The listing builds one solid part. Answer for the finished solid, in the listing's coordinates (mm). A direction names the side the tool comes from. Give positions to 0.01 mm unless a question says otherwise; leave off trailing zeros. Order: outer loops, then holes, each group sorted by start corner. A loop starts at its lowest first (then second) coordinate and runs counter-clockwise, first axis right, second up. Notation, with made-up numbers: M 53,-36 L 103,-36 A22 ccw 103,0 Z; hole C -25,22 d9. An arc over 180 degrees is marked long. Answer as a JSON object with one key per item and string values. Group by question number.
```python
from build123d import *

# Parameters (mm, degrees)
BOSS_EXTRUDE1_DEPTH = 6
CUT_EXTRUDE1_DEPTH  = 2.5
SKETCH3_R           = 1
CUT_EXTRUDE2_DEPTH  = 7
SKETCH4_R           = 2
CUT_EXTRUDE3_DEPTH  = 1.5
SKETCH5_R           = 1.25
CUT_EXTRUDE4_DEPTH  = 7


with BuildPart() as part:
    # Sketch1 → Boss-Extrude1 (new body)
    with BuildSketch(Plane.XY):
        with BuildLine():
            Line((0, 4.5), (23, 4.5))
            ThreePointArc((23, 4.5), (27.5, 0), (23, -4.5))
            Line((23, -4.5), (0, -4.5))
            ThreePointArc((0, -4.5), (-4.5, 0), (0, 4.5))
        make_face()
    extrude(amount=BOSS_EXTRUDE1_DEPTH)

    # Sketch2 → Cut-Extrude1 (cut)
    with BuildSketch(Plane.XY.offset(6)):
        with BuildLine():
            Line((2.115862708, 2.725), (15.116246568, 1.95))
            ThreePointArc((15.116246568, 1.95), (16.953461867, 0), (15.116246568, -1.95))
            Line((15.116246568, -1.95), (2.115862708, -2.725))
            ThreePointArc((2.115862708, -2.725), (-3.45, 0), (2.115862708, 2.725))
        make_face()
    extrude(amount=-CUT_EXTRUDE1_DEPTH, mode=Mode.SUBTRACT)

    # Sketch3 → Cut-Extrude2 (cut, through all)
    with BuildSketch(Plane.XY.offset(6)):
        Circle(SKETCH3_R)
    extrude(amount=-CUT_EXTRUDE2_DEPTH, mode=Mode.SUBTRACT)

    # Sketch4 → Cut-Extrude3 (cut)
    with BuildSketch(Plane(origin=(0, 0, 0), x_dir=(-1, 0, 0), z_dir=(0, 0, -1))):
        Circle(SKETCH4_R)
    extrude(amount=-CUT_EXTRUDE3_DEPTH, mode=Mode.SUBTRACT)

    # Sketch5 → Cut-Extrude4 (cut, through all)
    with BuildSketch(Plane.XY.offset(6)):
        with Locations((25, 0)):
            Circle(SKETCH5_R)
    extrude(amount=-CUT_EXTRUDE4_DEPTH, mode=Mode.SUBTRACT)


solid = part.part
```
Item 1: Consider probe 1 along X at (y, z) = (-0.5, 3.85); probe 2 along X at (y, z) = (-1, 5.75); probe 3 along Z at (x, y) = (6, 0.5). Determine where each line is inside the solid, lowest interval first. Write a range as from..to.
Item 2: Section C-C (x = 25) is taken. Determine the outline of the cut face in (y, z), and give its area (3 significant figures).
Item 3: Section A-A (y = 0) is taken. Determine the outline of the cut face in (x, z), and give its area (3 significant figures).
Item 4: A tool of negligible diameter and unlimited length cuts with its end or side. For faces 5 (the cylindrical face through (0, -1, 3)), 6 (the cylindrical face through (16.953, 0.041, 4.768)), 7 (the flat face through (-1, -1, 1.5)), from which of +Z, -Z, +X, -X, +Y, -Y can it reach the whole face along a straight path? Write none if from no direction.
Item 5: Flat-ended cylindrical pins translate along their axes: P1, Ø2, axis at x = 0.5, y = 0, coming from the -Z side; P2, Ø4, axis at x = 4, y = 0.5, coming from the +Z side; P3, Ø1.5, axis at y = 0.5, z = 3.5, coming from the -X side. Find the tip coordinate at first contact, or state that the pin passes through.
Item 6: Section D-D (x = 3) is taken. Determine the outline of the cut face in (y, z), and give its area (3 significant figures).
Item 7: Determine the mould class of faces 1 (the flat face through (12, -4.5, 3)), 2 (the cylindrical face through (26.155, -0.479, 3.042)), 3 (the cylindrical face through (-4.5, -0.1, 3)), 4 (the cylindrical face through (27.5, 0.1, 3)) for opening direction X: released by +X, released by -X, zero draft, split by the parting line, or undercut.
Item 8: Section B-B (z = 4.6) is taken. Determine the outline of the cut face in (x, y) (3 decimals).
Values found:
{
 "1": {"probe 1": "x = -4.47..-3.41, 16.89..23.85, 26.15..27.47", "probe 2": "x = -4.39..-3.3, 16.68..24.25, 25.75..27.39", "probe 3": "z = 0..3.5"},
 "2": {"outline": "M -4.03,0 L -1.25,0 L -1.25,6 L -4.03,6 Z; M 1.25,0 L 4.03,0 L 4.03,6 L 1.25,6 Z", "area": "33.4 mm^2"},
 "3": {"outline": "M -4.5,0 L -2,0 L -2,1.5 L -1,1.5 L -1,3.5 L -3.45,3.5 L -3.45,6 L -4.5,6 Z; M 1,1.5 L 2,1.5 L 2,0 L 23.75,0 L 23.75,6 L 16.95,6 L 16.95,3.5 L 1,3.5 Z; M 26.25,0 L 27.5,0 L 27.5,6 L 26.25,6 Z", "area": "116 mm^2"},
 "4": {"face 5": "+Z, -Z", "face 6": "+Z", "face 7": "-Z"},
 "5": {"P1": "stops at z = 1.5", "P2": "stops at z = 3.5", "P3": "stops at x = -4.5"},
 "6": {"outline": "M -4.5,0 L 4.5,0 L 4.5,6 L 2.67,6 L 2.67,3.5 L -2.67,3.5 L -2.67,6 L -4.5,6 Z", "area": "40.6 mm^2"},
 "7": {"face 1": "zero draft", "face 2": "undercut", "face 3": "released by -X", "face 4": "released by +X"},
 "8": {"outline": "M 0,-4.5 L 23,-4.5 A4.5 ccw 23,4.5 L 0,4.5 A4.5 ccw Z; hole M 2.116,-2.725 L 15.116,-1.95 A1.953 ccw 15.116,1.95 L 2.116,2.725 A3.45 ccw long Z; hole C 25,0 d2.5"}
}
